Job drawing, mm, ordinate dimensions from the low corner. One solid piece. Give positions to 0.01 mm unless a question says otherwise; leave off trailing zeros. Write each loop counter-clockwise with the first axis right and the second up, starting at its lowest first coordinate (ties: lowest second). Pieces come first, ordered by that corner, then holes. Notation, with made-up numbers: (74, 63.25) -> (79, 63.25) arc R19 ccw to (79, 69.25) -> close; hole circle Ø5 at (29.25, 66). An arc over 180 degrees is marked (long way). One line per question, with ' | ' between items. Start each with the question number.
(1) Pull direction Z, two halves, no side cores. Call the marked faces 1, 2 and 3: released by +Z, released by -Z, zero draft, split by the parting line, or undercut.
(2) Band-saw the part on B-B, the plane z = 16. Give the cut face in (x, y).
(3) Pin check, flat tips, straight feed: P1, Ø2, axis at x = 19, z = 25.5, coming from the -Y side; P2, Ø2, axis at x = 10.5, z = 28.5, coming from the -Y side; P3, Ø4, axis at x = 18, z = 30, coming from the -Y side; P4, Ø3, axis at x = 11.5, y = 2, coming from the +Z side. Stop position of each tip, or through.
(4) Drill centre lines: probe 1 along X at (y, z) = (5.5, 24) (1 decimal); probe 2 along X at (y, z) = (5.75, 20); probe 3 along Y at (x, z) = (19.5, 30.5). Where is each one in solid material? Low to high. Write a range as from..to.
(5) Band-saw the part on C-C, the plane z = 30. Give the cut face in (x, y).
(6) Band-saw the part on D-D, the plane x = 4. Give the cut face in (y, z), and give its area (3 significant figures).
(7) Band-saw the part on A-A, the plane x = 14. Give the cut face in (y, z) (1 decimal).
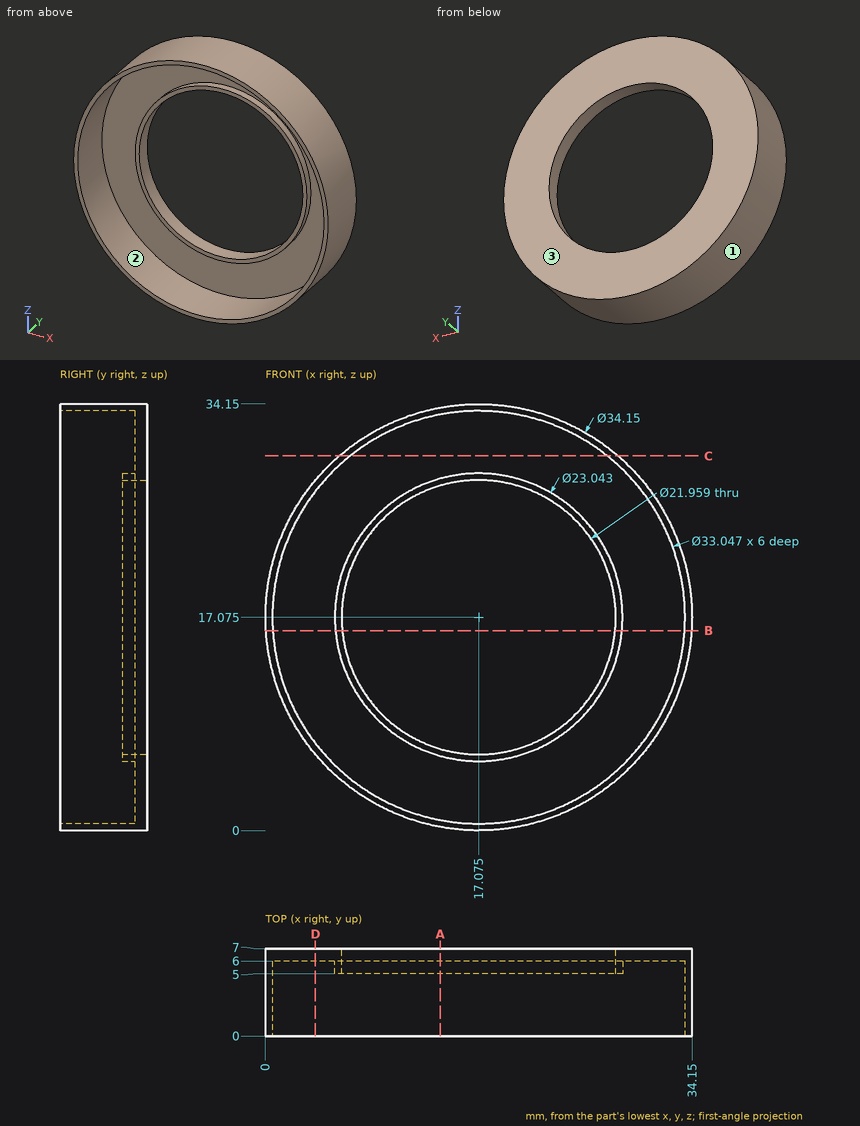
Results:
1) face 1: split by the parting line | face 2: undercut | face 3: zero draft
2) outline: (0.03, 0) -> (0.59, 0) -> (0.59, 6) -> (5.6, 6) -> (5.6, 5) -> (6.15, 5) -> (6.15, 7) -> (0.03, 7) -> close; (28, 5) -> (28.55, 5) -> (28.55, 6) -> (33.56, 6) -> (33.56, 0) -> (34.12, 0) -> (34.12, 7) -> (28, 7) -> close
3) P1: passes through | P2: stops at y = 6 | P3: stops at y = 5 | P4: stops at z = 33.66
4) probe 1: x = 1.5..2.1, 7.9..8.6, 25.6..26.3, 32.1..32.7 | probe 2: x = 0.25..0.81, 5.93..6.49, 27.66..28.22, 33.34..33.9 | probe 3: y = 6..7
5) outline: (5.92, 0) -> (6.78, 0) -> (6.78, 6) -> (27.37, 6) -> (27.37, 0) -> (28.23, 0) -> (28.23, 7) -> (5.92, 7) -> close
6) outline: (0, 6.09) -> (7, 6.09) -> (7, 28.06) -> (0, 28.06) -> (0, 27.18) -> (6, 27.18) -> (6, 6.97) -> (0, 6.97) -> close | area: 32.5 mm²
7) outline: (0, 0.3) -> (7, 0.3) -> (7, 6.5) -> (5, 6.5) -> (5, 6) -> (6, 6) -> (6, 0.8) -> (0, 0.8) -> close; (0, 33.3) -> (6, 33.3) -> (6, 28.2) -> (5, 28.2) -> (5, 27.6) -> (7, 27.6) -> (7, 33.9) -> (0, 33.9) -> close
